Check sheet for the modelled part. Datum: model origin and axes. Units: mm. Face numbers are marked on the shaded views. A direction names the side the tool comes from. Coordinates: 2 decimals unless noted, no trailing zeros. Loops run counter-clockwise (first coordinate to the right, second up) from the corner with the lowest first, then second, coordinate; pieces in that order, holes last. Notation, with made-up numbers: (35, -17) -> (59, -17) arc R11 ccw to (59, 4) -> close; hole circle Ø6 at (-32, -20.5). An arc over 180 degrees is marked (long way). Use one line per item in the form item = value.
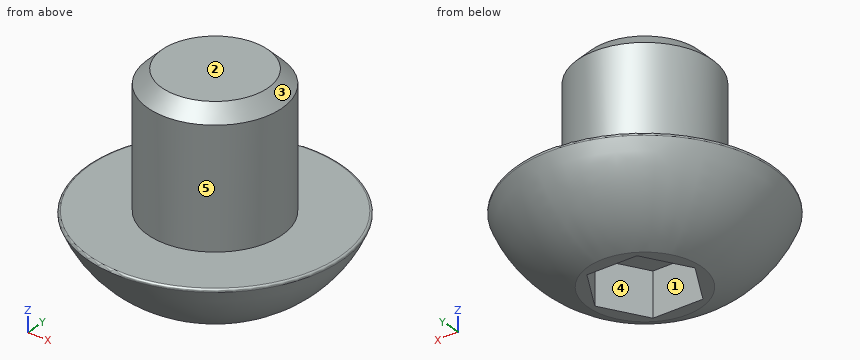
Autodesk Inventor part; units mm, degrees
ref_plane "YZ Plane" through (0, 0, 0) normal (1, 0, 0) x (0, 1, 0)
ref_plane "XZ Plane" through (0, 0, 0) normal (0, 1, 0) x (-1, 0, 0)
ref_plane "XY Plane" through (0, 0, 0) normal (0, 0, 1) x (1, 0, 0)
sketch "Sketch1" plane through (0, 0, 0) normal (0, 0, 1) x (1, 0, 0)
  circle A0 centre (0, 0) radius 2.413
  dimension "d0" = 4.826
extrude "Extrusion1" add sketch "Sketch1" along normal blind 4.7752
sketch "Sketch2" plane through (0, 0, 0) normal (0, 1, 0) x (-1, 0, 0)
  line L0 (0, 0) -> (0, -2.5654)
  line L1 (0, 0) -> (4.5085, 0)
  line L2 (0, -2.5654) -> (2.032, -2.5654)
  line L3 (4.5085, 0) -> (4.5085, 4.071) construction
  arc A0 (4.5791, -0.105) -> (4.5085, 0) centre (4.5085, -0.0762) ccw
  arc A1 (2.032, -2.5654) -> (4.5791, -0.105) centre (0.5168, 1.5517) ccw
  line L4 (4.5847, 0.6553) -> (4.5847, -0.0762) construction
  dimension "d3" = 2.5654
  dimension "d6" = 2.032
  dimension "d12" = 4.5847
  dimension "d18" = 0.0762
revolve "Revolution1" add sketch "Sketch2" angle 360 about axis through (0, 0, 0) along (0, 0, -1)
sketch "Sketch3" plane through (0, 0, -2.5654) normal (0, 0, -1) x (-1, 0, 0)
  circle A0 centre (0, 0) radius 2.032
  line L0 (-0.9165, 1.5875) -> (0.9165, 1.5875)
  line L1 (0.9165, 1.5875) -> (1.8331, 0)
  line L2 (1.8331, 0) -> (0.9165, -1.5875)
  line L3 (0.9165, -1.5875) -> (-0.9165, -1.5875)
  line L4 (-0.9165, -1.5875) -> (-1.8331, 0)
  line L5 (-1.8331, 0) -> (-0.9165, 1.5875)
  dimension "d8" = 3.175
extrude "Extrusion2" cut sketch "Sketch3" against normal blind 1.5875 contours L0 L1 L2 L3 L4 L5
chamfer "Chamfer1" distance 0.508 angle 45 1 edges at (-2.413, 0, 4.7752)
thread "Thread1"
properties part number "10-32 BHCS x375" material "Steel"
(1) Section check A-A, the plane z = 0.5. Record the boundary of the cut face in (x, y), plus the area to 3 significant figures.
Established:
outline = circle Ø4.83 at (0, 0)
area = 18.3 mm²
(2) Go/stop test with flat-tipped pins: P1, Ø2, axis at x = 2.5, z = -1, coming from the +Y side; P2, Ø3, axis at y = 3, z = -0.5, coming from the +X side; P3, Ø1.7, axis at x = -0.5, z = -1.5, coming from the +Y side; P4, Ø4.5, axis at x = 1.5, y = 2, coming from the +Z side. Record where each tip stops, or that it passes through.
Established:
P1 = 4.13
P2 = 4.31
P3 = 4.29
P4 = 4.78
(3) Mould release check, pull along X, two halves, no side actions. Record for the marked faces 1, 2 and 3: +X half, -X half, draft (parallel to the pull), parting line (faces both ways), or undercut.
Established:
face_1 = undercut
face_2 = draft
face_3 = parting line
(4) Tool access check on the marked faces 4 and 5. Record the directions out of +Z, -Z, +X, -X, +Y, -Y that give a thin tool (end or side, any length) a straight path to the whole face; none if there is none.
Established:
face_4 = -Z
face_5 = +Z
(5) Scan lines: line 1 along Y through (x, z) = (1.25, -1.25); line 2 along X through (y, z) = (-1.25, -2); line 3 along X through (y, z) = (2, 2). Record each from-to range of solid material in increasing order.
Established:
line_1 = -3.69 to -1.01, 1.01 to 3.69
line_2 = -2.83 to -1.11, 1.11 to 2.83
line_3 = -1.35 to 1.35
